```python
from build123d import *

# Parameters (mm, degrees)
F0_W     = 40
F0_H     = 20
F0_R     = 1.65
F1_DEPTH = 8
F2_SIZE  = 3
F3_R     = 2.55
F4_DEPTH = 20.001


with BuildPart() as f1:
    # F0 (on Right) → F1 (new body)
    with BuildSketch(Plane.YZ):
        Rectangle(F0_W, F0_H)
        with Locations((-12, 0)):
            Circle(F0_R, mode=Mode.SUBTRACT)
        with Locations((12, 0)):
            Circle(F0_R, mode=Mode.SUBTRACT)
    extrude(amount=F1_DEPTH)

    # F2
    f2_edges = [f1.edges().sort_by_distance(p)[0] for p in [
        (8, -13.65, 0),
        (8, 10.35, 0),
    ]]
    chamfer(f2_edges, length=F2_SIZE)

    # F3 (on face) → F4 (cut, through all)
    with BuildSketch(Plane(origin=(0, 0, -10), x_dir=(1, 0, 0), z_dir=(0, 0, -1))):
        with Locations((4, 0)):
            Circle(F3_R)
    extrude(amount=-F4_DEPTH, mode=Mode.SUBTRACT)


solid = f1.part
```
Geometry check sheet. Reference: the model listing, model coordinates, mm. Coordinates: 2 decimals unless noted, no trailing zeros. Order: outer loops, then holes, each group sorted by start corner. A loop starts at its lowest first (then second) coordinate and runs counter-clockwise, first axis right, second up. Notation, with made-up numbers: (40, 4.5) - (95, 4.5) arc R21 ccw to (95, 20.5) - close; hole circle Ø10 at (-1.5, 42). An arc over 180 degrees is marked (long way). Answer as a JSON object with one key per item and string values. Group by question number.
Item 1: Sectioned sample at D-D, the plane x = 0.75. Record the cut outline in (y, z), and give its area (3 significant figures).
Item 2: Scan lines: probe 1 along Y at (x, z) = (4, 4); probe 2 along Y at (x, z) = (5.75, 1.25); probe 3 along Z at (x, y) = (1.4, -12). Record each from-to range of solid material in increasing order.
Item 3: Sectioned sample at A-A, the plane x = 4. Record the cut outline in (y, z).
Item 4: Draft check along Y on faces 1 (the face through (5.19, -10.3, -0.7)), 2 (the face through (4, 20, 0)), 3 (the face through (4, -20, 0)), 4 (the face through (0, 0, 0)). Enter one of: +Y half, -Y half, draft (parallel to the pull), parting line (faces both ways), or undercut.
Item 5: Sectioned sample at C-C, the plane y = -12. Record the cut outline in (x, z).
Item 6: Sectioned sample at B-B, the plane z = 0. Record the cut outline in (x, y).
Resolved:
{
 "1": {"outline": "(-20, -10) - (20, -10) - (20, 10) - (-20, 10) - close; hole circle Ø3.3 at (-12, 0); hole circle Ø3.3 at (12, 0)", "area": "783 mm^2"},
 "2": {"probe 1": "-20 to -2.55, 2.55 to 20", "probe 2": "-20 to -14.05, -9.95 to -1.85, 1.85 to 9.95, 14.05 to 20", "probe 3": "-10 to -1.65, 1.65 to 10"},
 "3": {"outline": "(-20, -10) - (-2.55, -10) - (-2.55, 10) - (-20, 10) - close; (2.55, -10) - (20, -10) - (20, 10) - (2.55, 10) - close; hole circle Ø3.3 at (-12, 0); hole circle Ø3.3 at (12, 0)"},
 "4": {"face 1": "undercut", "face 2": "+Y half", "face 3": "-Y half", "face 4": "draft"},
 "5": {"outline": "(0, -10) - (8, -10) - (8, -4.65) - (5, -1.65) - (0, -1.65) - close; (0, 1.65) - (5, 1.65) - (8, 4.65) - (8, 10) - (0, 10) - close"},
 "6": {"outline": "(0, -20) - (8, -20) - (8, -16.65) - (5, -13.65) - (0, -13.65) - close; (0, -10.35) - (5, -10.35) - (8, -7.35) - (8, 7.35) - (5, 10.35) - (0, 10.35) - close; (0, 13.65) - (5, 13.65) - (8, 16.65) - (8, 20) - (0, 20) - close; hole circle Ø5.1 at (4, 0)"}
}
